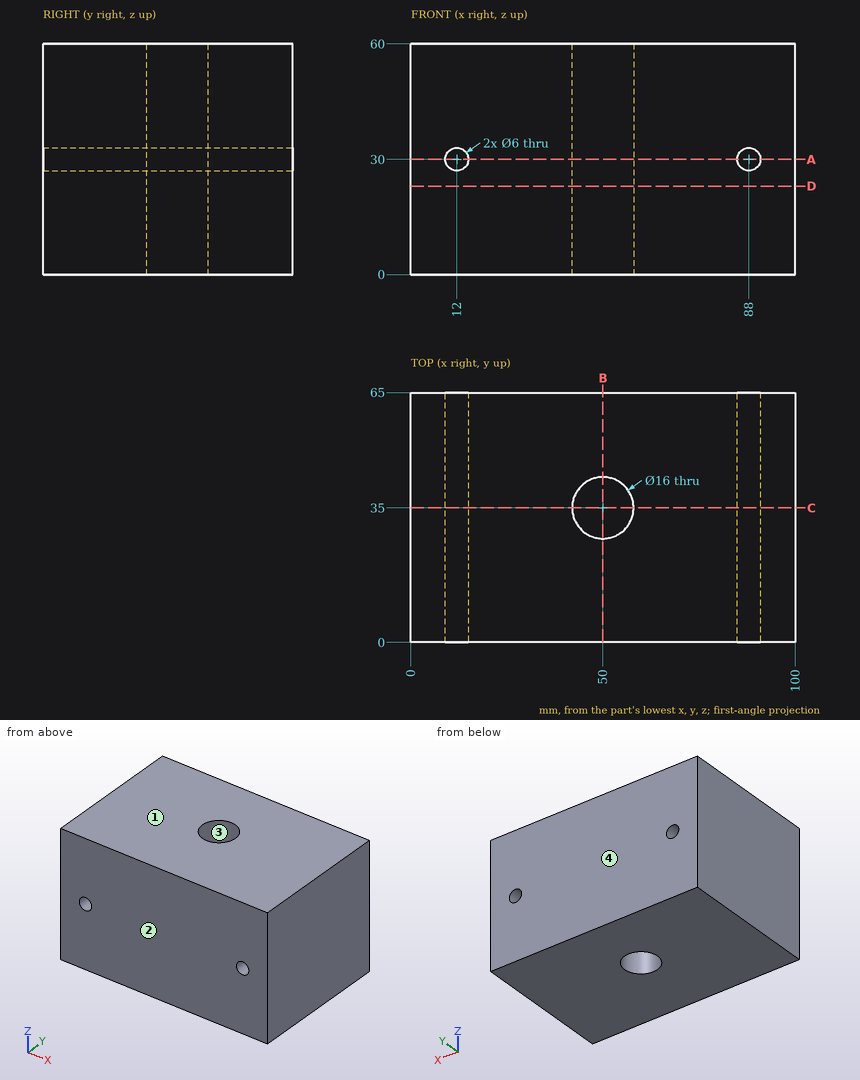
Answer from the drawing. Dimensions are ordinates in mm from the lowest x, y and z of the part. Give positions to 0.01 mm unless a question says otherwise; leave off trailing zeros. Order: outer loops, then holes, each group sorted by start corner. A loop starts at its lowest first (then second) coordinate and runs counter-clockwise, first axis right, second up. Notation, with made-up numbers: (45.5, 66) -> (62.5, 66) arc R17 cw to (62.5, 73) -> close; hole circle Ø10 at (-8, -8). An arc over 180 degrees is marked (long way). One line per item, written item: value. Start each with the question number.
(1) Straight lines are drawn through the part: L1, parallel to X at y = 22, z = 30; L2, parallel to X at y = 32, z = 30; L3, parallel to Z at x = 88, y = 21. For each, find the intervals that lie inside material, in ascending order.
(2) The part is cut by section A-A (z = 30). Determine the outline of the cut face in (x, y), and give its area (3 significant figures).
(3) The part is cut by section D-D (z = 23). Determine the outline of the cut face in (x, y).
(4) The part is cut by section C-C (y = 35). Determine the outline of the cut face in (x, z).
(5) The part is cut by section B-B (x = 50). Determine the outline of the cut face in (y, z).
(6) Flat-ended cylindrical pins translate along their axes: P1, Ø8, axis at y = 45.5, z = 45, coming from the -X side; P2, Ø3.5, axis at x = 12, z = 30, coming from the -Y side. Find the tip coordinate at first contact, or state that the pin passes through.
(7) For a pull along Y with two mould halves and no side action, classify the marked faces 1, 2, 3 and 4 as released by +Y, released by -Y, zero draft, split by the parting line, or undercut.
Taken from the geometry:
1. L1: 0 to 9, 15 to 85, 91 to 100
1. L2: 0 to 9, 15 to 42.58, 57.42 to 85, 91 to 100
1. L3: 0 to 27, 33 to 60
2. outline: (0, 0) -> (9, 0) -> (9, 65) -> (0, 65) -> close; (15, 0) -> (85, 0) -> (85, 65) -> (15, 65) -> close; (91, 0) -> (100, 0) -> (100, 65) -> (91, 65) -> close; hole circle Ø16 at (50, 35)
2. area: 5,520 mm^2
3. outline: (0, 0) -> (100, 0) -> (100, 65) -> (0, 65) -> close; hole circle Ø16 at (50, 35)
4. outline: (0, 0) -> (42, 0) -> (42, 60) -> (0, 60) -> close; (58, 0) -> (100, 0) -> (100, 60) -> (58, 60) -> close; hole circle Ø6 at (12, 30); hole circle Ø6 at (88, 30)
5. outline: (0, 0) -> (27, 0) -> (27, 60) -> (0, 60) -> close; (43, 0) -> (65, 0) -> (65, 60) -> (43, 60) -> close
6. P1: x = 0
6. P2: through
7. face 1: zero draft
7. face 2: released by -Y
7. face 3: undercut
7. face 4: released by +Y
